Verification items for this drawing (mm, ordinates from the low corner). Give positions to 0.01 mm unless a question says otherwise; leave off trailing zeros. Loops run counter-clockwise (first coordinate to the right, second up) from the corner with the lowest first, then second, coordinate; pieces in that order, holes last. Notation, with made-up numbers: M 55,71 L 82,71 A19 cw 82,77 Z; hole C -25,45 d5. An arc over 180 degrees is marked long. Answer in a Markdown table with one row per item.
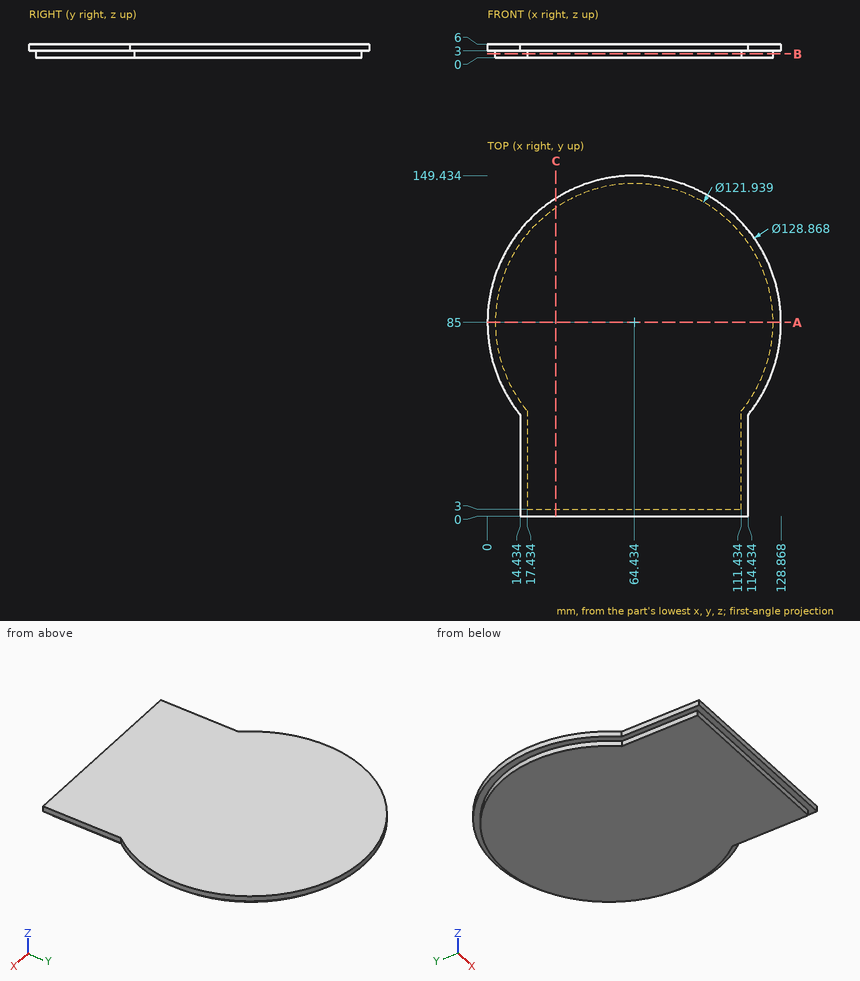
Item 1: Scan lines: L1, parallel to Z at x = 16, y = 17; L2, parallel to X at y = 28, z = 4.15; L3, parallel to Y at x = 123, z = 4.8 (1 decimal). Record each from-to range of solid material in increasing order. Write a range as [from, to].
Reported:
| item | result |
|---|---|
| L1 | z = [3, 6] |
| L2 | x = [14.43, 114.43] |
| L3 | y = [58.1, 111.9] |
Item 2: Sectioned sample at B-B (z = 1.65). Record the cut outline in (x, y), and give its area (3 significant figures).
Reported:
| item | result |
|---|---|
| outline | M 17.43,3 L 111.43,3 L 111.43,46.16 A60.97 ccw long 17.43,46.16 Z |
| area | 14,300 mm^2 |
Item 3: Sectioned sample at C-C (x = 30). Record the cut outline in (y, z) (1 decimal).
Reported:
| item | result |
|---|---|
| outline | M 0,3 L 3,3 L 3,0 L 135.3,0 L 135.3,3 L 139.5,3 L 139.5,6 L 0,6 Z |
Item 4: Sectioned sample at A-A (y = 85). Record the cut outline in (x, z) (1 decimal).
Reported:
| item | result |
|---|---|
| outline | M 0,3 L 3.5,3 L 3.5,0 L 125.4,0 L 125.4,3 L 128.9,3 L 128.9,6 L 0,6 Z |
Item 5: Go/stop test with flat-tipped pins: pin 1 (0.9 mm diameter, centred on y = 33, z = 4.5, fed in from +X); pin 2 (1.5 mm diameter, centred on x = 94.5, z = 4.5, fed in from +Y); pin 3 (1.5 mm diameter, centred on x = 73, z = 1, fed in from -Y). Record where each tip stops, or that it passes through.
Reported:
| item | result |
|---|---|
| pin 1 | stops at x = 114.43 |
| pin 2 | stops at y = 142.38 |
| pin 3 | stops at y = 3 |
